Could you check a few things on this model? Use its own coordinates, in mm. A direction names the side the tool comes from. Round coordinates to 2 decimals unless told otherwise and drop trailing zeros. Write each loop counter-clockwise with the first axis right and the second up, starting at its lowest first coordinate (ties: lowest second). Pieces come first, ordered by that corner, then holes. Notation, with made-up numbers: (88.5, 25.5) -> (113.5, 25.5) arc R21 cw to (113.5, 38.5) -> close; hole circle Ø8 at (-12.75, -38). An arc over 180 degrees is marked (long way). Answer as CSV lines item,"result". Start each with the question number.
Q1. Will these pins go through, and if not, where does the flat tip stop? pin 1 Ø1 at (x, z) = (-47.5, -14) entering from -Y; pin 2 Ø5 at (y, z) = (2.5, -30.5) entering from -X; pin 3 Ø1 at (y, z) = (53, -31) entering from +X.
Q2. Imagine slicing it at A-A on y = -78. Please give me the cut outline in (x, z), and give its area (3 significant figures).
Q3. If we mould it in two halves opening along Y, with no side actions, what happens to faces 3 (the flat face through (-31.9, -105.931, -42.4)), 4 (the cylindrical face through (42.04, 31.31, -24.05)), 5 (the flat face through (-21, -16, -3))? For each: pulls with the +Y half, pulls with the -Y half, needs draft (parallel to the pull), parting line crosses it, or undercut.
Q4. Imagine slicing it at D-D on y = 6. Please give me the cut outline in (x, z), and give its area (3 significant figures).
Q5. For faces 1 (the flat face through (-21, 74.069, -22)), 2 (the flat face through (-21, 71.069, -22)), which set-ups out of +Z, -Z, +X, -X, +Y, -Y let a thin tool reach every point of the face, with its end or its side?
Q6. If I drill on line 1 (Z direction, x = 20.5, y = 12.5); line 2 (X direction, y = -36, z = -11); line 3 (Y direction, x = -33, z = -7), over which ranges is the centre line in solid material (lowest first)? Write a range as [from, to].
Q7. Imagine slicing it at B-B on x = -34. Please give me the cut outline in (y, z).
Q8. Imagine slicing it at C-C on z = -26.5. Please give me the cut outline in (x, y).
from build123d import *

# Parameters (mm, degrees)
F0_W     = 155.25
F0_H     = 180
F1_DEPTH = 45
F2_SIZE2 = 80
F2_SIZE  = 30
F3_SIZE2 = 30
F3_SIZE  = 80
F4_T     = -3
F6_D     = 3.175


with BuildPart() as f1:
    # F0 (on Top) → F1 (new body)
    with BuildSketch(Plane.XY):
        with Locations((-19.9909230247, -15.9310551924)):
            Rectangle(F0_W, F0_H)
    extrude(amount=-F1_DEPTH)

    # F2
    f2_edges = [f1.edges().sort_by_distance(p)[0] for p in [
        (-97.615923, 74.068945, -22.5),
    ]]
    f2_side = f1.faces().sort_by_distance((-19.990923, 74.068945, -22.5))[0]
    chamfer(f2_edges, length=F2_SIZE, length2=F2_SIZE2, reference=f2_side)

    # F3
    f3_edges = [f1.edges().sort_by_distance(p)[0] for p in [
        (57.634077, 74.068945, -22.5),
    ]]
    f3_side = f1.faces().sort_by_distance((57.634077, -15.931055, -22.5))[0]
    chamfer(f3_edges, length=F3_SIZE, length2=F3_SIZE2, reference=f3_side)

    # F4
    f4_openings = [f1.faces().sort_by_distance(p)[0] for p in [
        (-19.990923, -105.931055, -22.5),
    ]]
    offset(amount=F4_T, openings=f4_openings)

    # F6 (through all)
    with Locations(Plane(origin=(48.5785698877, 18.2169637079, 0), x_dir=(-0.3511234416, 0.9363291776, 0), z_dir=(0.9363291776, 0.3511234416, 0))):
        with Locations((14.2099045093, -22.5)):
            Hole(F6_D / 2)


solid = f1.part
Checks:
1,pin 1,"y = 71.07"
1,pin 2,"x = -95.39"
1,pin 3,"x = 35.72"
2,outline,"(-97.62, -45) -> (57.63, -45) -> (57.63, 0) -> (-97.62, 0) -> close; hole (-94.62, -42) -> (54.63, -42) -> (54.63, -3) -> (-94.62, -3) -> close"
2,area,"1,170 mm^2"
3,face 3,"pulls with the -Y half"
3,face 4,"undercut"
3,face 5,"needs draft"
4,outline,"(-93.14, -45) -> (53.16, -45) -> (53.16, 0) -> (-93.14, 0) -> close; hole (-89.94, -42) -> (49.96, -42) -> (49.96, -3) -> (-89.94, -3) -> close"
4,area,"1,130 mm^2"
5,face 1,"+Z, -Z, +X, -X, +Y"
5,face 2,"-Y"
6,line 1,"[-45, -42], [-3, 0]"
6,line 2,"[-97.62, -94.62], [54.63, 57.63]"
6,line 3,"[71.07, 74.07]"
7,outline,"(-105.93, -45) -> (74.07, -45) -> (74.07, 0) -> (-105.93, 0) -> (-105.93, -3) -> (71.07, -3) -> (71.07, -42) -> (-105.93, -42) -> close"
8,outline,"(-97.62, -105.93) -> (-94.62, -105.93) -> (-94.62, -6.48) -> (-65.54, 71.07) -> (25.56, 71.07) -> (54.63, -6.48) -> (54.63, -105.93) -> (57.63, -105.93) -> (57.63, -5.93) -> (27.63, 74.07) -> (-67.62, 74.07) -> (-97.62, -5.93) -> close"
